Input: part model. Units: mm. Frame: model coordinates. A direction names the side the tool comes from. Give positions to 0.01 mm unless a question says otherwise; leave off trailing zeros. Loops run counter-clockwise (first coordinate to the right, second up) from the corner with the lowest first, then second, coordinate; pieces in that order, holes last. Notation, with made-up numbers: M 67.5,1.25 L 79.5,1.25 A26 cw 79.5,27.25 Z; hole C 53.25,36.5 d3. An arc over 180 degrees is marked long. One line per item, written item: value. Start each with the question number.
(1) Section B-B on z = 3. Output: boundary loops of the cut face in (x, y).
(2) Section A-A on y = 3.5. Output: boundary loops of the cut face in (x, z), plus the area to 3 significant figures.
(3) Pin query (flat end, axial travel): P1, Ø1, axis at y = -5, z = 5, coming from the -X side; P2, Ø2, axis at x = 6.5, z = 3.5, coming from the +Y side; P3, Ø2, axis at x = 0, z = 6.5, coming from the +Y side. Return the tip coordinate at first contact, or that it passes through.
(4) Section C-C on y = -7.25. Output: boundary loops of the cut face in (x, z).
(5) Ray query, line 1 along Z through (x, y) = (8, -3); line 2 along X through (y, z) = (0.75, 4.5); line 3 along Z through (x, y) = (9, -10.25). Return the intervals inside material, ascending. Write a range as from..to.
(6) Access query for faces 5 (the cylindrical face through (9.845, -10.958, 3.012)), 6 (the flat face through (11.43, -4.805, 3.944)), 7 (the cylindrical face through (6.78, -4.71, 0.55)). Directions: +Z, -Z, +X, -X, +Y, -Y. A direction counts if a zero-diameter tool reaches every point of the face in a straight line with its end or side. Return the directions, or none.
(7) Section D-D on x = -3. Output: boundary loops of the cut face in (y, z).
(8) Pull-direction query (Y, two-part tool) for faces 1 (the flat face through (7, -14, 1)), 2 (the flat face through (3.6, -4.84, 3.94)), 3 (the cylindrical face through (-3.802, -4.641, 3.944)), 4 (the flat face through (7.9, -3.2, 8)); classes: released by +Y, released by -Y, zero draft, split by the parting line, or undercut.
```python
from build123d import *

# Parameters (mm, degrees)
F1_DEPTH = 8
F2_R     = 1.5
F3_DEPTH = 25
F2_R_2   = 2.5
F4_DEPTH = 6
F6_START = -2
F5_R     = 3.5
F6_DEPTH = 23


with BuildPart() as f1:
    # F0 (on Top) → F1 (new body)
    with BuildSketch(Plane.XY):
        with BuildLine():
            ThreePointArc((-6.4197371813, 4.7735704167), (-7.5946658073, 2.5141700966), (-8, 0))
            ThreePointArc((-8, 0), (-5.6568542495, -5.6568542495), (0, -8))
            ThreePointArc((0, -8), (4.6410709926, -6.5161691231), (7.5605008751, -2.6151150104))
            Line((7.5605008751, -2.6151150104), (3.3365949124, -4.9866957387))
            ThreePointArc((3.3365949124, -4.9866957387), (-3.8856695712, -4.5718237044), (-5.4593337085, 2.4891113795))
            Line((-5.4593337085, 2.4891113795), (-6.4197371813, 4.7735704167))
        make_face()
        with BuildLine():
            ThreePointArc((7.5605008751, -2.6151150104), (4.6410709926, -6.5161691231), (0, -8))
            Line((0, -8), (15.1210017502, -8))
            ThreePointArc((15.1210017502, -8), (10.4799307576, -6.5161691231), (7.5605008751, -2.6151150104))
        make_face()
        with BuildLine():
            Line((12.1655220018, -5.2216031501), (7.5605008751, -2.6151150104))
            ThreePointArc((7.5605008751, -2.6151150104), (10.4799307576, -6.5161691231), (15.1210017502, -8))
            ThreePointArc((15.1210017502, -8), (20.7778559997, -5.6568542495), (23.1210017502, 0))
            ThreePointArc((23.1210017502, 0), (22.79183999, 2.2711760607), (21.8314415756, 4.3554560439))
            Line((21.8314415756, 4.3554560439), (20.5803354587, 2.4891113795))
            ThreePointArc((20.5803354587, 2.4891113795), (20.9842773813, 1.2735771962), (21.1210017502, 0))
            ThreePointArc((21.1210017502, 0), (18.1431798977, -5.1832846001), (12.1655220018, -5.2216031501))
        make_face()
        with BuildLine():
            ThreePointArc((21.8314415756, 4.3554560439), (22.79183999, 2.2711760607), (23.1210017502, 0))
            Line((23.1210017502, 0), (26.0024620047, 5.1898341576))
            Line((26.0024620047, 5.1898341576), (23.510556668, 6.8602855317))
            Line((23.510556668, 6.8602855317), (21.8314415756, 4.3554560439))
        make_face()
        with BuildLine():
            Line((-10.1314789225, 5.8615841737), (-8, 0))
            ThreePointArc((-8, 0), (-7.5946658073, 2.5141700966), (-6.4197371813, 4.7735704167))
            Line((-6.4197371813, 4.7735704167), (-7.3659350164, 7.0242392831))
            Line((-7.3659350164, 7.0242392831), (-10.1314789225, 5.8615841737))
        make_face()
    extrude(amount=F1_DEPTH)

    # F2 (on face) → F3 (cut)
    with BuildSketch(Plane.XZ.offset(8)):
        with Locations((7.5357314199, 3.9691259153)):
            Circle(F2_R)
    extrude(amount=-F3_DEPTH, mode=Mode.SUBTRACT)

    # F2 (on face) → F4 (join)
    with BuildSketch(Plane.XZ.offset(8)):
        with BuildLine():
            ThreePointArc((8.031755077, 0), (10.5344056793, 1.3218721145), (11.5357314199, 3.9691259153))
            ThreePointArc((11.5357314199, 3.9691259153), (4.8884776191, 6.9678001747), (7.0397077629, 0))
            Line((7.0397077629, 0), (8.031755077, 0))
        make_face()
        with Locations((7.5357314199, 3.9691259153)):
            Circle(F2_R_2, mode=Mode.SUBTRACT)
    extrude(amount=F4_DEPTH)

    # F5 (on face) → F6 (cut)
    with BuildSketch(Plane.XZ.offset(8).offset(F6_START)):
        with Locations((7.5357314199, 3.9691259153)):
            Circle(F5_R)
    extrude(amount=-F6_DEPTH, mode=Mode.SUBTRACT)


solid = f1.part
```
Output values:
1. outline: M -10.13,5.86 L -8,0 A8 ccw 0,-8 L 3.65,-8 L 3.65,-14 L 5.23,-14 L 5.23,-8 L 6.39,-8 L 6.39,-6 L 4.17,-6 L 4.17,-4.52 L 3.34,-4.99 A6 cw -5.46,2.49 L -7.37,7.02 Z; M 8.68,-8 L 9.84,-8 L 9.84,-14 L 11.42,-14 L 11.42,-8 L 15.12,-8 A8 ccw 23.12,0 L 26,5.19 L 23.51,6.86 L 20.58,2.49 A6 cw 12.17,-5.22 L 10.9,-4.5 L 10.9,-6 L 8.68,-6 Z
2. outline: M -9.27,0 L -5.88,0 L -5.88,8 L -9.27,8 Z; M 21.26,0 L 25.06,0 L 25.06,8 L 21.26,8 Z
2. area: 57.6 mm²
3. P1: stops at x = -6.61
3. P2: stops at y = -6
3. P3: stops at y = -5.92
4. outline: M -3.38,0 L 18.5,0 L 18.5,8 L -3.38,8 Z; hole C 7.54,3.97 d3
5. line 1: z = 0..0.5, 7.44..8
5. line 2: x = -8.27..-5.95, 21.07..23.54
5. line 3: z = 0.25..1.94, 6..7.69
6. face 5: -Y
6. face 6: +Z, -Z, +Y
6. face 7: +Y
7. outline: M -7.42,0 L -5.2,0 L -5.2,8 L -7.42,8 Z
8. face 1: released by -Y
8. face 2: released by +Y
8. face 3: undercut
8. face 4: zero draft
